For this review, take the finished solid that the model builds, in its own axes (mm). A direction names the side the tool comes from. Give positions to 0.01 mm unless a question says otherwise; leave off trailing zeros. Write each loop counter-clockwise with the first axis right and the second up, starting at its lowest first coordinate (ties: lowest second). Pieces come first, ordered by that corner, then holes.
from build123d import *

# Parameters (mm, degrees)
F0_W     = 177.8
F0_H     = 91.44
F0_W_2   = 38.1
F0_H_2   = 38.1
F1_DEPTH = 25.4
F2_W     = 5.08
F2_H     = 5.08
F3_DEPTH = 6.35


with BuildPart() as f1:
    # F0 (on Top) → F1 (new body)
    with BuildSketch(Plane.XY):
        with Locations((-0.942165, 55.466111)):
            Rectangle(F0_W, F0_H)
        with Locations((-65.712165, 33.876111)):
            Rectangle(F0_W_2, F0_H_2, mode=Mode.SUBTRACT)
        with Locations((-22.532165, 33.876111)):
            Rectangle(F0_W_2, F0_H_2, mode=Mode.SUBTRACT)
        with Locations((20.647835, 33.876111)):
            Rectangle(F0_W_2, F0_H_2, mode=Mode.SUBTRACT)
        with Locations((63.827835, 33.876111)):
            Rectangle(F0_W_2, F0_H_2, mode=Mode.SUBTRACT)
        with Locations((-65.712165, 77.056111)):
            Rectangle(F0_W_2, F0_H_2, mode=Mode.SUBTRACT)
        with Locations((-22.532165, 77.056111)):
            Rectangle(F0_W_2, F0_H_2, mode=Mode.SUBTRACT)
        with Locations((20.647835, 77.056111)):
            Rectangle(F0_W_2, F0_H_2, mode=Mode.SUBTRACT)
        with Locations((63.827835, 77.056111)):
            Rectangle(F0_W_2, F0_H_2, mode=Mode.SUBTRACT)
    extrude(amount=F1_DEPTH)

    # F2 (on face) → F3 (join)
    with BuildSketch(Plane.XY.offset(25.4)):
        with Locations((-87.302165, 98.646111)):
            Rectangle(F2_W, F2_H)
        with Locations((-87.302165, 12.286111)):
            Rectangle(F2_W, F2_H)
        with Locations((85.417835, 12.286111)):
            Rectangle(F2_W, F2_H)
        with Locations((85.417835, 98.646111)):
            Rectangle(F2_W, F2_H)
    extrude(amount=F3_DEPTH)


solid = f1.part
(1) The part is to be moulded in two halves that separate along Y. For faces 5 (the flat face through (-87, 96.106, 29)), 6 (the flat face through (82.878, 12, 29)), say which applies: +Y half, -Y half, draft (parallel to the pull), parting line (faces both ways), or undercut.
(2) Clearance check with a flat-ended pin moving along its axis: pin 1 Ø12 at (x, y) = (34.5, 84) entering from +Z. State where the tip first meets the part, or that it passes through.
(3) For L1, parallel to Y at x = 54.5, z = 11; L2, parallel to X at y = 68.5, z = 19.5; L3, parallel to Z at x = -45.5, y = 65, list the stretches that pass through material, from the lowest coordinate up.
(4) We need section A-A (x = -26). Write out the cut boundary in (y, z), and give its area (3 significant figures).
(5) Tool access review of faces 1 (the flat face through (44.778, 77, 13)), 2 (the flat face through (-89.842, 55, 12)), 3 (the flat face through (-84.762, 12, 29)), 4 (the flat face through (85, 96.106, 29)): name each direction out of +Z, -Z, +X, -X, +Y, -Y from which nothing blocks a thin tool from reaching the whole face with its end or side.
(6) We need section C-C (z = 5). Count the separate pieces of the cut face and the enclosed holes in it, and give its area (3 significant figures).
(7) We need section B-B (y = 48). Write out the cut boundary in (x, z).
The answers:
1. face 5: undercut
1. face 6: draft
2. pin 1: stops at z = 25.4
3. L1: y = 9.75 to 14.83, 52.93 to 58.01, 96.11 to 101.19
3. L2: x = -89.84 to -84.76, -46.66 to -41.58, -3.48 to 1.6, 39.7 to 44.78, 82.88 to 87.96
3. L3: z = 0 to 25.4
4. outline: (9.75, 0) - (14.83, 0) - (14.83, 25.4) - (9.75, 25.4) - close; (52.93, 0) - (58.01, 0) - (58.01, 25.4) - (52.93, 25.4) - close; (96.11, 0) - (101.19, 0) - (101.19, 25.4) - (96.11, 25.4) - close
4. area: 387 mm2
5. face 1: +Z, -Z
5. face 2: +Z, -Z, -X, +Y, -Y
5. face 3: +Z, +Y, -Y
5. face 4: +Z, +X, -X
6. separate pieces: 1
6. enclosed holes: 8
6. area: 4,650 mm2
7. outline: (-89.84, 0) - (-84.76, 0) - (-84.76, 25.4) - (-89.84, 25.4) - close; (-46.66, 0) - (-41.58, 0) - (-41.58, 25.4) - (-46.66, 25.4) - close; (-3.48, 0) - (1.6, 0) - (1.6, 25.4) - (-3.48, 25.4) - close; (39.7, 0) - (44.78, 0) - (44.78, 25.4) - (39.7, 25.4) - close; (82.88, 0) - (87.96, 0) - (87.96, 25.4) - (82.88, 25.4) - close
